Read the model definition and answer for the solid it produces. Units are mm, in the model's axes. A direction names the side the tool comes from. Coordinates: 2 decimals unless noted, no trailing zeros. Order: outer loops, then holes, each group sorted by start corner. A loop starts at its lowest first (then second) coordinate and runs counter-clockwise, first axis right, second up. Notation, with made-up numbers: M -35.5,26.5 L 21.5,26.5 A19 ccw 21.5,61.5 Z; hole C 42.5,-12 d8. An arc over 180 degrees is marked long. Put each result on its own line as item: value.
Autodesk Inventor part; units mm, degrees
ref_plane "YZ Plane" through (0, 0, 0) normal (1, 0, 0) x (0, 1, 0)
ref_plane "XZ Plane" through (0, 0, 0) normal (0, 1, 0) x (-1, 0, 0)
ref_plane "XY Plane" through (0, 0, 0) normal (0, 0, 1) x (1, 0, 0)
sketch "スケッチ1" plane through (0, 0, 0) normal (0, 0, 1) x (1, 0, 0)
  circle A0 centre (0, 0) radius 6.25
  line L0 (0, 13) -> (-16, 13)
  line L1 (-16, 13) -> (-16, -13)
  line L2 (-16, -13) -> (0, -13)
  line L3 (0, -13) -> (0, 13)
  line L4 (0, 13) -> (3, 13)
  line L5 (3, 13) -> (3, -13)
  line L6 (3, -13) -> (0, -13)
  line L7 (0, -13) -> (0, 13)
  point P0 (-16, 0)
  point P1 (3, -5.4829)
  point P2 (3, 5.4829)
  dimension "d0" = 12.5
  dimension "d1" = 16
  dimension "d2" = 26
  dimension "d3" = 3
extrude "プレート1" add sketch "スケッチ1" along normal blind 1.5 contours A0 L3 L4 L5 | L5 L6 L3 A0 | A0 L3 L2 L1 L0
sketch "スケッチ2" plane through (-14.5, 13, 1.5) normal (-1, 0, 0) x (0, -1, 0)
  line L0 (26, 0) -> (0, 0)
  line L1 (0, 0) -> (0, -11)
  line L2 (0, -11) -> (26, -11)
  line L3 (26, -11) -> (26, 0)
edge flange "フランジ1" height 11 angle 90 thickness 1.5 bend radius 1.5 thickness toward (-1, 0, 0) relief tear relief width 1.5 relief depth 0.75 edges at (-16, 0, 0) wall of the first edge with corners at (-14.5, -13, 1.5) (-14.5, 13, 1.5) (-14.5, 13, -9.5) (-14.5, -13, -9.5)
bend "曲げ1"
corner "コーナー1"
sketch "スケッチ3" plane through (-16, -13, -9.5) normal (-1, 0, 0) x (0, 0, 1)
  line L0 (8, 0) -> (0, 0)
  line L1 (0, 0) -> (8, 0)
  line L2 (8, 0) -> (8, -26)
  line L3 (8, -26) -> (0, -26)
  line L4 (0, -26) -> (0, 0)
  line L5 (8, 0) -> (8, 26)
  arc A0 (0, 0) -> (3, 26) centre (-111.1667, 26) ccw
  line L6 (3, 20) -> (3, 26) construction
  line L7 (0, 26) -> (8, 26)
  line L8 (0, 0) -> (0, 26)
  point P0 (9.5, 13)
  point P1 (8, 0)
  dimension "d15" = 26
  dimension "d21" = 5
sheet face with bend "面2" sketch "スケッチ3" thickness 1.5 toward (1, 0, 0) bend radius 1.5 contours L2 L3 L4 L0
bend "曲げ2"
extrude "切り取り1" cut sketch "スケッチ3" against normal blind 1.5 contours L8 L7 A0
sketch "スケッチ5" plane through (0, 0, 0) normal (0, 0, -1) x (-1, 0, 0)
  circle A0 centre (0, 10.5) radius 0.85
  circle A1 centre (0, -10.5) radius 0.85
  point P0 (0, 0)
extrude "切り取り2" cut sketch "スケッチ5" against normal blind 1.5
sketch "スケッチ6" plane through (-16, -39, -1.5) normal (-1, 0, 0) x (0, 0, 1)
  circle A0 centre (-5, 23.5) radius 0.85
  circle A1 centre (-5, 2.5) radius 0.85
  point P0 (1.5, 39)
extrude "切り取り3" cut sketch "スケッチ6" against normal blind 1.5
equation "\"d23\" = Thickness"
equation "\"d25\" = Thickness"
equation "\"d27\" = Thickness"
equation "\"d4\" = Thickness"
equation "\"d5\" = BendReliefWidth"
equation "\"d6\" = BendReliefDepth"
equation "\"d7\" = MinimumRemnant"
equation "\"d8\" = TransitionRadius"
equation "\"d11\" = BendRadius"
equation "\"d12\" = CornerReliefSize"
equation "\"d13\" = GapSize"
equation "\"d14\" = JacobiRadiusSize"
equation "\"d16\" = BendRadius"
equation "\"d17\" = BendReliefWidth"
equation "\"d19\" = MinimumRemnant"
equation "\"d18\" = BendReliefDepth"
equation "\"d20\" = TransitionRadius"
equation "\"BendRadius\" = Thickness"
equation "\"BendReliefWidth\" = Thickness"
equation "\"BendReliefDepth\" = 0.5 * Thickness"
equation "\"CornerReliefSize\" = 4 * Thickness"
equation "\"MinimumRemnant\" = 2 * Thickness"
equation "\"TransitionRadius\" = BendRadius"
equation "\"JacobiRadiusSize\" = BendRadius"
equation "\"GapSize\" = Thickness"
properties part number "hipjoint_toleg_under_right"
Q1. Consider line 1 along Y through (x, z) = (0, 0.65); line 2 along Z through (x, y) = (-12.5, -3); line 3 along Y through (x, z) = (-3, 1.25). Determine where each line is inside the solid, lowest interval first.
Answers below:
line 1: y = -13 to -11.35, -9.65 to -6.25, 6.25 to 9.65, 11.35 to 13
line 2: z = 0 to 1.5
line 3: y = -13 to -5.48, 5.48 to 13
Q2. Find section B-B on x = -5. Write down the section's boundary in (y, z).
Answers below:
outline: M -13,0 L -3.75,0 L -3.75,1.5 L -13,1.5 Z; M 3.75,0 L 13,0 L 13,1.5 L 3.75,1.5 Z
Q3. Find section C-C on z = 0.5. Write down the section's boundary in (x, y).
Answers below:
outline: M -15.24,-13 L 3,-13 L 3,-5.48 A6.25 cw long 3,5.48 L 3,13 L -15.24,13 Z; hole C 0,-10.5 d1.7; hole C 0,10.5 d1.7
Q4. Find section A-A on y = -15.5. Write down the section's boundary in (x, z), plus the area to 3 significant figures.
Answers below:
outline: M -16,-9.5 L -14.5,-9.5 L -14.5,-7.35 L -16,-7.35 Z; M -16,-5.65 L -14.5,-5.65 L -14.5,-1.5 L -16,-1.5 Z
area: 9.45 mm^2
Q5. For a pull along Y with two mould halves and no side action, classify faces 4 (the face through (-15, -39, -5)), 5 (the face through (-6.247, -0.181, 0.74)), 6 (the face through (-15.14, 0.18, 0.6)) as +Y half, -Y half, draft (parallel to the pull), parting line (faces both ways), or undercut.
Answers below:
face 4: -Y half
face 5: undercut
face 6: draft
Q6. Given pin 1 (1.5 mm diameter, centred on x = -7.5, z = 0.5, fed in from -Y); pin 2 (1.2 mm diameter, centred on x = -15, y = -23, fed in from +Z); pin 3 (6.5 mm diameter, centred on y = -7.5, z = -6, fed in from +X), each flat-ended and moving along its own axis, determine where each tip first touches the part or whether it passes through.
Answers below:
pin 1: stops at y = -13
pin 2: stops at z = -1.5
pin 3: stops at x = -14.5
Q7. Find section D-D on y = -4. Write down the section's boundary in (x, z), plus the area to 3 significant figures.
Answers below:
outline: M -16,-7.77 L -14.5,-7.77 L -14.5,-1.5 A1.5 cw -13,0 L -4.8,0 L -4.8,1.5 L -13,1.5 A3 ccw -16,-1.5 Z
area: 27.0 mm^2
Q8. A tool of negligible diameter and unlimited length cuts with its end or side. For faces 1 (the face through (0.111, 11.343, 0.74)), 2 (the face through (-7, 0, 0)), 3 (the face through (-15, -26, -1.5)), from which of +Z, -Z, +X, -X, +Y, -Y can it reach the whole face along a straight path? Write none if from no direction.
Answers below:
face 1: +Z, -Z
face 2: -Z, +X, +Y, -Y
face 3: +Z, +X, -X, -Y
